Geometry: final body of the model. Coordinates: model frame, mm. Give positions to 0.01 mm unless a question says otherwise; leave off trailing zeros. Write each loop counter-clockwise with the first axis right and the second up, starting at its lowest first coordinate (ties: lowest second). Pieces come first, ordered by that corner, then holes.
```python
from build123d import *

# Parameters (mm, degrees)
SKETCH1_R           = 3.2639
BOSS_EXTRUDE1_DEPTH = 3.175
CAVITY1_OUTLINE_W   = 11.43
CAVITY1_OUTLINE_H   = 18.479477922
FILLET2_R           = 1.27


# Read off the part's stored shape, not the designer's step: Cavity1
with BuildPart() as part:
    # Sketch1 → Boss-Extrude1 (new body)
    with BuildSketch(Plane.XY):
        with BuildLine():
            ThreePointArc((8.804991066, 1.226471495), (0, 8.89), (-8.804991066, 1.226471495))
            Line((-8.804991066, 1.226471495), (-15.875, -49.53))
            Line((-15.875, -49.53), (15.875, -49.53))
            Line((15.875, -49.53), (8.804991066, 1.226471495))
        make_face()
        Circle(SKETCH1_R, mode=Mode.SUBTRACT)
    extrude(amount=BOSS_EXTRUDE1_DEPTH)

    # Cavity1 outline → Cavity1 (revolve, cut)
    with BuildSketch(Plane(origin=(5.822510153, -48.093039184, -8.961753145), x_dir=(0.8468434564524782, -0.1362359794546486, 0.5140971874710584), z_dir=(0, 0.9666347575686124, 0.2561586333900735))):
        with Locations((5.715, -12.145132975)):
            Rectangle(CAVITY1_OUTLINE_W, CAVITY1_OUTLINE_H)
    revolve(axis=Axis((5.822510153, -48.093039184, -8.961753145), (0.5318422324934529, 0.21692626250019303, -0.818588319226507)), mode=Mode.SUBTRACT)

    # Fillet2
    # the kernel refuses this fillet: 1.27 mm, written as the material it takes off along each edge
    with BuildSketch(Plane(origin=(-15.875, -49.53, -3.64790796), x_dir=(0.13796079814219978, 0.990437690203663, 0), z_dir=(0, 0, 1))) as fillet2_piece_1:
        with BuildLine():
            CenterArc((FILLET2_R * 1.14894738902, -FILLET2_R), FILLET2_R, 90, 97.929863559)
            Line((FILLET2_R * 0.158509698812, -FILLET2_R * 1.13796079814), (0, 0))
            Line((0, 0), (FILLET2_R * 1.14894738902, 0))
        make_face()
    extrude(amount=10.47081592, mode=Mode.SUBTRACT)
    with BuildSketch(Plane(origin=(15.875, -49.53, -3.64790796), x_dir=(-0.1379607981421991, 0.9904376902036632, 0), z_dir=(0, 0, 1))) as fillet2_piece_2:
        with BuildLine():
            CenterArc((FILLET2_R * 1.14894738902, FILLET2_R), FILLET2_R, 172.070136441, 97.929863559)
            Line((FILLET2_R * 0.158509698812, FILLET2_R * 1.13796079814), (0, 0))
            Line((0, 0), (FILLET2_R * 1.14894738902, 0))
        make_face()
    extrude(amount=10.47081592, mode=Mode.SUBTRACT)


solid = part.part
```
Item 1: Section A-A, the plane y = -2.5. Return the cut outline in (x, z) (3 decimals), plus the area to 3 significant figures.
Found:
outline: (-9.324, 0) - (-2.098, 0) - (-2.098, 3.175) - (-9.324, 3.175) - close; (2.098, 0) - (9.324, 0) - (9.324, 3.175) - (2.098, 3.175) - close
area: 45.9 mm2
Item 2: Section C-C, the plane y = -36. Return the cut outline in (x, z) (3 decimals), plus the area to 3 significant figures.
Found:
outline: (-13.99, 0) - (13.99, 0) - (13.99, 3.175) - (-13.99, 3.175) - close
area: 88.8 mm2
Item 3: Line query: L1, parallel to X at y = -41.5, z = 2.3; L2, parallel to Y at x = 0, z = 0.9; L3, parallel to Y at x = 0, z = 1.15. Output: solid intervals per line, ascending.
Found:
L1: x = -14.76 to -7.87, 7.96 to 14.76
L2: y = -38.94 to -3.26, 3.26 to 8.89
L3: y = -38.99 to -3.26, 3.26 to 8.89
Item 4: Section B-B, the plane y = -27.5. Return the cut outline in (x, z) (3 decimals).
Found:
outline: (-12.806, 0) - (12.806, 0) - (12.806, 3.175) - (-12.806, 3.175) - close
